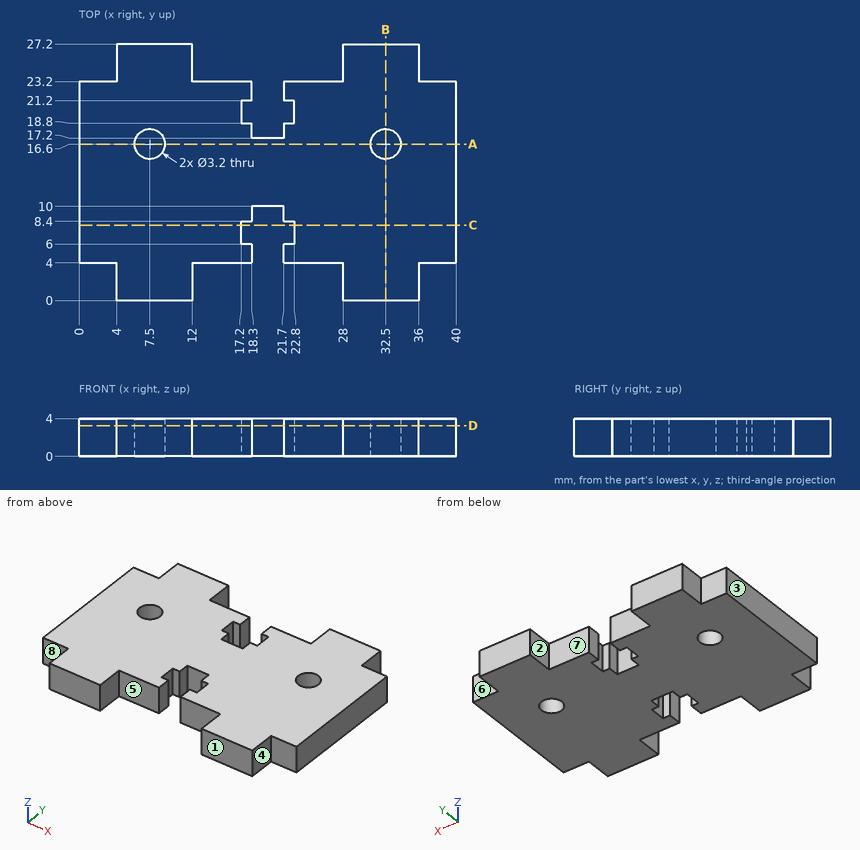
Geometry: see drawing. Coordinates: mm, zero at the bounding-box minimum. A direction names the side the tool comes from. Coordinates: 2 decimals unless noted, no trailing zeros. Write each loop counter-clockwise with the first axis right and the second up, starting at its lowest first coordinate (ties: lowest second). Pieces come first, ordered by that corner, then holes.
1) Section B-B on x = 32.5. Output: boundary loops of the cut face in (y, z), and give its area (3 significant figures).
2) Section C-C on y = 8. Output: boundary loops of the cut face in (x, z).
3) Material intervals for line 1 along X through (y, z) = (3.25, 2.5); line 2 along X through (y, z) = (22.5, 3); line 3 along Y through (x, z) = (7.5, 1.1), sorted ascending.
4) Set-up query: the marked faces 5, 6, 7 and 8. Return all of +Z, -Z, +X, -X, +Y, -Y with unobstructed straight access to the full face (end or side cutting, diameter ignored); none if empty.
5) Section A-A on y = 16.6. Output: boundary loops of the cut face in (x, z).
6) Mould query, pull axis X, two halves, no side actions, for the marked faces 1, 2, 3 and 4. Classes: pulls with the +X half, pulls with the -X half, needs draft (parallel to the pull), parting line crosses it, or undercut.
7) Pin query (flat end, axial travel): pin 1 Ø1.6 at (y, z) = (4.5, 2.5) entering from -X; pin 2 Ø0.6 at (x, z) = (17.5, 2) entering from -Y; pin 3 Ø1.7 at (x, z) = (20.5, 2.5) entering from -Y; pin 4 Ø2 at (y, z) = (24.5, 2.5) entering from +X. Return the tip coordinate at first contact, or that it passes through.
8) Section D-D on z = 3.25. State how many separate pieces and enclosed holes the cut face has, and give its area (3 significant figures).
Check result:
1. outline: (0, 0) - (15, 0) - (15, 4) - (0, 4) - close; (18.2, 0) - (27.2, 0) - (27.2, 4) - (18.2, 4) - close
1. area: 96.0 mm2
2. outline: (0, 0) - (17.2, 0) - (17.2, 4) - (0, 4) - close; (22.8, 0) - (40, 0) - (40, 4) - (22.8, 4) - close
3. line 1: x = 4 to 12, 28 to 36
3. line 2: x = 0 to 18.3, 21.7 to 40
3. line 3: y = 0 to 15, 18.2 to 27.2
4. face 5: +Z, -Z, -Y
4. face 6: +Z, -Z, +X, +Y
4. face 7: +Z, -Z, +Y
4. face 8: +Z, -Z, -X, -Y
5. outline: (0, 0) - (5.9, 0) - (5.9, 4) - (0, 4) - close; (9.1, 0) - (30.9, 0) - (30.9, 4) - (9.1, 4) - close; (34.1, 0) - (40, 0) - (40, 4) - (34.1, 4) - close
6. face 1: needs draft
6. face 2: undercut
6. face 3: pulls with the -X half
6. face 4: pulls with the +X half
7. pin 1: stops at x = 0
7. pin 2: stops at y = 4
7. pin 3: stops at y = 10
7. pin 4: stops at x = 36
8. separate pieces: 1
8. enclosed holes: 2
8. area: 829 mm2
